from build123d import *
from OCP.BRepAlgoAPI import BRepAlgoAPI_Cut
from OCP.TopTools import TopTools_ListOfShape
from build123d.topology import SkipClean

# Parameters (mm, degrees)
BOSS_EXTRUDE1_DEPTH            = 40
CUT_EXTRUDE1_DEPTH             = 9
CUT_EXTRUDE2_DEPTH             = 8
CUT_EXTRUDE3_DEPTH             = 9
CUT_EXTRUDE4_DEPTH             = 8
CUT_EXTRUDE5_DEPTH             = 8
CUT_EXTRUDE6_DEPTH             = 8
CUT_EXTRUDE7_DEPTH             = 40.73
F_7_0_7_DIAMETER_HOLE1_D       = 7
F_7_0_7_DIAMETER_HOLE1_DEPTH   = 29
F_13_0_13_DIAMETER_HOLE1_D     = 13
F_13_0_13_DIAMETER_HOLE1_DEPTH = 29


with BuildPart() as part:
    # Sketch1 → Boss-Extrude1 (new body)
    with BuildSketch(Plane(origin=(0, 20, 0), x_dir=(1, 0, 0), z_dir=(0, 1, 0))):
        with BuildLine():
            Line((563.96485174, 507.513718698), (563.96485174, 562.736423486))
            Line((563.96485174, 562.736423486), (554.690781869, 562.894803628))
            ThreePointArc((554.690781869, 562.894803628), (545.704943994, 565.795150829), (539.853906856, 573.206133263))
            Line((539.853906856, 573.206133263), (522.524343645, 610.429990226))
            ThreePointArc((522.524343645, 610.429990226), (512.649800976, 621.543175495), (497.931198247, 623.634159339))
            Line((497.931198247, 623.634159339), (399.830947056, 608.608698386))
            ThreePointArc((399.830947056, 608.608698386), (385.610832142, 608.137408426), (371.923585817, 612.02238853))
            Line((371.923585817, 612.02238853), (95.310746964, 771.494097008))
            add(Edge.make_bspline(
                [(60.287007155, 752.902507236), (59.408683029, 762.769524202), (58.560960325, 776.204376236), (76.94287295, 783.298520304), (86.753146937, 776.493697586), (95.310746964, 771.494097008)],
                knots=[0, 0, 0, 0, 0.5, 0.5, 1, 1, 1, 1], degree=3))
            ThreePointArc((60.287007155, 752.902507236), (112.407005996, 551.803928099), (202.762947005, 364.739937083))
            ThreePointArc((202.762947005, 364.739937083), (207.132055784, 361.391783138), (212.632195034, 361.173346422))
            Line((212.632195034, 361.173346422), (367.65464082, 417.084401042))
            ThreePointArc((367.65464082, 417.084401042), (380.966681082, 418.419109504), (394.090964942, 415.82198883))
            Line((394.090964942, 415.82198883), (660.231475403, 329.574923038))
            ThreePointArc((660.231475403, 329.574923038), (670.878462163, 333.606992627), (669.266978502, 344.877264703))
            Line((669.266978502, 344.877264703), (553.73117364, 453.239940989))
            ThreePointArc((553.73117364, 453.239940989), (543.342125743, 483.300566911), (563.96485174, 507.513718698))
        make_face()
    extrude(amount=-BOSS_EXTRUDE1_DEPTH)

    # Sketch2 → Cut-Extrude1 (cut)
    with BuildSketch(Plane(origin=(0, 20, 0), x_dir=(-1, 0, 0), z_dir=(0, 1, 0))):
        with BuildLine():
            Line((-375.961047941, -499.395283579), (-375.961047941, -501.895283579))
            Line((-375.961047941, -501.895283579), (-380.19743869, -501.895283579))
            ThreePointArc((-380.19743869, -501.895283579), (-383.334721276, -503.261242071), (-385.264615119, -506.086820662))
            Line((-385.264615119, -506.086820662), (-385.264615119, -565.732528297))
            ThreePointArc((-385.264615119, -565.732528297), (-383.334721277, -568.558106887), (-380.197438694, -569.924065379))
            Line((-380.197438694, -569.924065379), (-375.961047941, -569.924065379))
            Line((-375.961047941, -569.924065379), (-375.961047941, -572.424065379))
            ThreePointArc((-375.961047941, -572.424065379), (-374.057242019, -577.020259457), (-369.461047941, -578.924065379))
            Line((-369.461047941, -578.924065379), (-361.195765613, -578.924065379))
            ThreePointArc((-361.195765613, -578.924065379), (-356.599571535, -577.020259457), (-354.695765613, -572.424065379))
            Line((-354.695765613, -572.424065379), (-354.695765613, -569.924065379))
            Line((-354.695765613, -569.924065379), (-350.459374862, -569.924065379))
            ThreePointArc((-350.459374862, -569.924065379), (-347.322092956, -568.55810734), (-345.3922012, -565.732528296))
            Line((-345.3922012, -565.732528296), (-345.3922012, -506.086820663))
            ThreePointArc((-345.3922012, -506.086820663), (-347.322092957, -503.261241618), (-350.459374866, -501.895283579))
            Line((-350.459374866, -501.895283579), (-354.695765613, -501.895283579))
            Line((-354.695765613, -501.895283579), (-354.695765613, -499.395283579))
            ThreePointArc((-354.695765613, -499.395283579), (-356.599571535, -494.799089501), (-361.195765613, -492.895283579))
            Line((-361.195765613, -492.895283579), (-369.461047941, -492.895283579))
            ThreePointArc((-369.461047941, -492.895283579), (-374.057242019, -494.799089501), (-375.961047941, -499.395283579))
        make_face()
    extrude(amount=-CUT_EXTRUDE1_DEPTH, mode=Mode.SUBTRACT)

    # Sketch3 → Cut-Extrude2 (cut)
    with BuildSketch(Plane(origin=(0, 11, 0), x_dir=(-1, 0, 0), z_dir=(0, 1, 0))):
        with BuildLine():
            Line((-361.195765613, -492.895279984), (-369.461047941, -492.895279984))
            ThreePointArc((-369.461047941, -492.895279984), (-374.057242019, -494.799085907), (-375.961047941, -499.395279985))
            Line((-375.961047941, -499.395279985), (-375.961047941, -501.895279985))
            ThreePointArc((-375.961047941, -501.895279985), (-374.057242221, -506.491473573), (-369.461048632, -508.395279293))
            Line((-369.461048632, -508.395279293), (-361.19104863, -508.395279293))
            ThreePointArc((-361.19104863, -508.395279293), (-356.596520928, -506.491186012), (-354.695765613, -501.895276389))
            Line((-354.695765613, -501.895276389), (-354.695765613, -499.395279984))
            ThreePointArc((-354.695765613, -499.395279984), (-356.599571535, -494.799085907), (-361.195765613, -492.895279984))
        make_face()
    extrude(amount=-CUT_EXTRUDE2_DEPTH, mode=Mode.SUBTRACT)

    # Sketch4 → Cut-Extrude3 (cut)
    with BuildSketch(Plane(origin=(0, 20, 0), x_dir=(-1, 0, 0), z_dir=(0, 1, 0))):
        with BuildLine():
            Line((-479.744131485, -572.424065379), (-479.744131485, -569.924065379))
            Line((-479.744131485, -569.924065379), (-475.507740734, -569.924065379))
            ThreePointArc((-475.507740734, -569.924065379), (-472.370458828, -568.55810734), (-470.440567072, -565.732528296))
            Line((-470.440567072, -565.732528296), (-470.440567072, -506.086820663))
            ThreePointArc((-470.440567072, -506.086820663), (-472.370458829, -503.261241618), (-475.507740738, -501.895283579))
            Line((-475.507740738, -501.895283579), (-479.744131485, -501.895283579))
            Line((-479.744131485, -501.895283579), (-479.744131485, -499.395283579))
            ThreePointArc((-479.744131485, -499.395283579), (-481.647937407, -494.799089501), (-486.244131485, -492.895283579))
            Line((-486.244131485, -492.895283579), (-494.509413812, -492.895283579))
            ThreePointArc((-494.509413812, -492.895283579), (-499.10560789, -494.799089501), (-501.009413812, -499.395283579))
            Line((-501.009413812, -499.395283579), (-501.009413812, -501.895283579))
            Line((-501.009413812, -501.895283579), (-505.245804562, -501.895283579))
            ThreePointArc((-505.245804562, -501.895283579), (-508.383087148, -503.261242071), (-510.312980991, -506.086820662))
            Line((-510.312980991, -506.086820662), (-510.312980991, -565.732528297))
            ThreePointArc((-510.312980991, -565.732528297), (-508.383087149, -568.558106887), (-505.245804566, -569.924065379))
            Line((-505.245804566, -569.924065379), (-501.009413812, -569.924065379))
            Line((-501.009413812, -569.924065379), (-501.009413812, -572.424065379))
            ThreePointArc((-501.009413812, -572.424065379), (-499.10560789, -577.020259457), (-494.509413812, -578.924065379))
            Line((-494.509413812, -578.924065379), (-486.244131485, -578.924065379))
            ThreePointArc((-486.244131485, -578.924065379), (-481.647937407, -577.020259457), (-479.744131485, -572.424065379))
        make_face()
    extrude(amount=-CUT_EXTRUDE3_DEPTH, mode=Mode.SUBTRACT)

    # Sketch5 → Cut-Extrude4 (cut)
    with BuildSketch(Plane(origin=(0, 11, 0), x_dir=(-1, 0, 0), z_dir=(0, 1, 0))):
        with BuildLine():
            Line((-486.244131485, -492.895283579), (-494.509413812, -492.895283579))
            ThreePointArc((-494.509413812, -492.895283579), (-499.10560789, -494.799089501), (-501.009413812, -499.395283579))
            Line((-501.009413812, -499.395283579), (-501.009413812, -501.895283579))
            ThreePointArc((-501.009413812, -501.895283579), (-499.108657916, -506.491191283), (-494.514131485, -508.395283579))
            Line((-494.514131485, -508.395283579), (-486.244131485, -508.395283579))
            ThreePointArc((-486.244131485, -508.395283579), (-481.647937407, -506.491477657), (-479.744131485, -501.895283579))
            Line((-479.744131485, -501.895283579), (-479.744131485, -499.395283579))
            ThreePointArc((-479.744131485, -499.395283579), (-481.647937407, -494.799089501), (-486.244131485, -492.895283579))
        make_face()
    extrude(amount=-CUT_EXTRUDE4_DEPTH, mode=Mode.SUBTRACT)


with BuildPart() as cut_extrude5_tool:
    # Sketch6 → Cut-Extrude5 (new body)
    with BuildSketch(Plane(origin=(0, 11, 0), x_dir=(-1, 0, 0), z_dir=(0, 1, 0))):
        with BuildLine():
            Line((-369.461049324, -578.924068974), (-361.195766995, -578.924068974))
            ThreePointArc((-361.195766995, -578.924068974), (-356.599572918, -577.020263051), (-354.695766995, -572.424068974))
            Line((-354.695766995, -572.424068974), (-354.695766995, -569.924072568))
            ThreePointArc((-354.695766995, -569.924072568), (-356.59652231, -565.328162946), (-361.191050012, -563.424069665))
            Line((-361.191050012, -563.424069665), (-369.461050015, -563.424069665))
            ThreePointArc((-369.461050015, -563.424069665), (-374.057243604, -565.327875385), (-375.961049323, -569.924068973))
            Line((-375.961049323, -569.924068973), (-375.961049323, -572.424068974))
            ThreePointArc((-375.961049323, -572.424068974), (-374.057243401, -577.020263051), (-369.461049324, -578.924068974))
        make_face()
    extrude(amount=-CUT_EXTRUDE5_DEPTH)


with BuildPart() as part_1:
    add(part.part)

    # Cut-Extrude5: cut by cut_extrude5_tool, with a tolerance
    cut_extrude5_stock = TopTools_ListOfShape()
    cut_extrude5_stock.Append(part_1.part.wrapped)
    cut_extrude5_tools = TopTools_ListOfShape()
    cut_extrude5_tools.Append(cut_extrude5_tool.part.wrapped)
    cut_extrude5_cut = BRepAlgoAPI_Cut()
    cut_extrude5_cut.SetArguments(cut_extrude5_stock)
    cut_extrude5_cut.SetTools(cut_extrude5_tools)
    cut_extrude5_cut.SetFuzzyValue(0.00001)
    cut_extrude5_cut.Build()
    add(Compound.cast(cut_extrude5_cut.Shape()).solids(), mode=Mode.REPLACE)

    # Sketch7 → Cut-Extrude6 (cut)
    with SkipClean():  # the faces are left unmerged after this step: merging them gives an invalid solid
        with BuildSketch(Plane(origin=(0, 11, 0), x_dir=(-1, 0, 0), z_dir=(0, 1, 0))):
            with BuildLine():
                Line((-494.509413812, -578.924065379), (-486.244131485, -578.924065379))
                ThreePointArc((-486.244131485, -578.924065379), (-481.647937407, -577.020259457), (-479.744131485, -572.424065379))
                Line((-479.744131485, -572.424065379), (-479.744131485, -569.924065379))
                ThreePointArc((-479.744131485, -569.924065379), (-481.647937407, -565.327871301), (-486.244131485, -563.424065379))
                Line((-486.244131485, -563.424065379), (-494.514131485, -563.424065379))
                ThreePointArc((-494.514131485, -563.424065379), (-499.108657916, -565.328157675), (-501.009413812, -569.924065379))
                Line((-501.009413812, -569.924065379), (-501.009413812, -572.424065379))
                ThreePointArc((-501.009413812, -572.424065379), (-499.10560789, -577.020259457), (-494.509413812, -578.924065379))
            make_face()
        extrude(amount=-CUT_EXTRUDE6_DEPTH, mode=Mode.SUBTRACT)

    # Sketch8 → Cut-Extrude7 (cut)
    with SkipClean():  # the faces are left unmerged after this step: merging them gives an invalid solid
        with BuildSketch(Plane.XY.offset(-514.76642324)):
            Polygon((463.964851744, -16), (563.964851744, -16), (563.964851744, 20), (513.964851744, 20), (513.964851744, 10), (463.964851744, 10), align=None)
        extrude(amount=-CUT_EXTRUDE7_DEPTH, mode=Mode.SUBTRACT)

    # Ø7.0 (7) Diameter Hole1
    with Locations(Plane(origin=(0, 20, 0), x_dir=(1, 0, 0), z_dir=(0, 1, 0))):
        with Locations((308.179113698, 575.311111117), (316.876935056, 502.297353485)):
            Hole(F_7_0_7_DIAMETER_HOLE1_D / 2, depth=F_7_0_7_DIAMETER_HOLE1_DEPTH)

    # Ø13.0 (13) Diameter Hole1
    with Locations(Plane(origin=(0, 20, 0), x_dir=(1, 0, 0), z_dir=(0, 1, 0))):
        with Locations((274.335910331, 496.233480955), (274.335910331, 579.213058938)):
            Hole(F_13_0_13_DIAMETER_HOLE1_D / 2, depth=F_13_0_13_DIAMETER_HOLE1_DEPTH)


solid = part_1.part
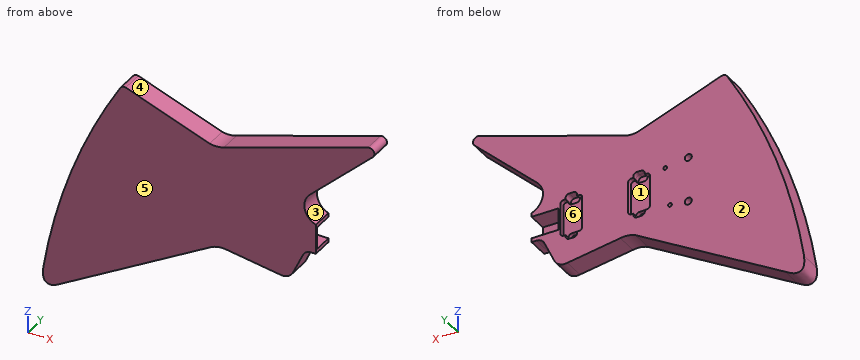
The listing builds one solid part. Answer for the finished solid, in the listing's coordinates (mm). Face numbers are marked on the shaded views. A direction names the side the tool comes from. Coordinates: 2 decimals unless noted, no trailing zeros. Write each loop counter-clockwise with the first axis right and the second up, starting at its lowest first coordinate (ties: lowest second). Pieces come first, ordered by that corner, then holes. Notation, with made-up numbers: (-27, -23.5) - (27, -23.5) arc R21 cw to (27, 9.5) - close; hole circle Ø8 at (-1, -14.5). An arc over 180 degrees is marked (long way). Return JSON: item names as keys, results as strings.
1. Which of the six approach directions +Z, -Z, +X, -X, +Y, -Y give full straight-line access (tool end or side, diameter ignored) to the marked faces 4, 5 and 6?
Final values:
{"face 4": "+Z, +Y, -Y", "face 5": "+Z, -Z, +X, -X, -Y", "face 6": "+Y"}
2. The part is cut by section C-C on x = 152. Determine the outline of the cut face in (y, z).
Final values:
{"outline": "(-20, -738.81) - (20, -738.81) - (20, -458.11) - (-20, -458.11) - close"}
3. Each of these flat-tipped pins is pushed along its axis until it touches: pin 1 Ø1.2 at (y, z) = (15.5, -571) entering from -X; pin 2 Ø6 at (y, z) = (0.5, -385) entering from -X; pin 3 Ø10 at (y, z) = (17, -525) entering from +X. Where does it stop, or does it pass through?
Final values:
{"pin 1": "x = 105.36", "pin 2": "x = 188.97", "pin 3": "x = 513.96"}
4. The part is cut by section D-D on x = 293. Determine the outline of the cut face in (y, z), then the cut area to 3 significant figures.
Final values:
{"outline": "(-20, -657.52) - (20, -657.52) - (20, -390.16) - (-20, -390.16) - close", "area": "10,700 mm^2"}
5. The part is cut by section A-A on z = -388. Determine the outline of the cut face in (x, y), then the cut area to 3 significant figures.
Final values:
{"outline": "(188.97, -20) - (287.01, -20) - (287.01, 20) - (188.97, 20) - close; (479.94, -20) - (623.29, -20) - (623.29, 20) - (479.94, 20) - close", "area": "9,660 mm^2"}
6. The part is cut by section B-B on z = -538.5. Determine the outline of the cut face in (x, y), then the cut area to 3 significant figures.
Final values:
{"outline": "(117.39, -20) - (563.96, -20) - (563.96, -16) - (463.96, -16) - (463.96, 10) - (513.96, 10) - (513.96, 20) - (510.31, 20) - (510.31, 11) - (470.44, 11) - (470.44, 20) - (385.26, 20) - (385.26, 11) - (345.39, 11) - (345.39, 20) - (117.39, 20) - close", "area": "14,000 mm^2"}
7. For a pull along X with two mould halves and no side action, classify the marked faces 1, 2 and 3 as +X half, -X half, draft (parallel to the pull), parting line (faces both ways), or undercut.
Final values:
{"face 1": "undercut", "face 2": "draft", "face 3": "+X half"}
8. Consider line 1 along X through (y, z) = (0, -578.5); line 2 along Z through (x, y) = (530, -2.5); line 3 along Z through (x, y) = (484, -10.5). Determine where each line is inside the solid, lowest interval first.
Final values:
{"line 1": "103.01 to 267.88, 280.8 to 306.74, 309.62 to 537.39", "line 2": "-594.37 to -555.5, -514.77 to -371.78", "line 3": "-621.5 to -555.5, -514.77 to -386.69"}
